```python
from build123d import *

# Parameters (mm, degrees)
F2_DEPTH = 40
F6_DEPTH = 40.001
F7_DEPTH = 40.001


with BuildPart() as f2:
    # F1 (on face) → F2 (new body)
    with BuildSketch(Plane.XY):
        Polygon((-30.25273, 38.586084), (-30.25273, 0), (-26.359774, 0), (-20, 11.340041), (-20, 0), (-10, 0), (-10, 11.340041), (0, 11.340041), (0, 0), (9.197158, 0), (9.197158, 11.045149), (13.475588, 0), (26.648319, 0), (34.74727, 11.808881), (34.74727, 38.586084), align=None)
        Polygon((-26.625307, 52.630479), (-42.740828, 52.770232), (-42.740828, 0), (-30.25273, 0), (-30.25273, 38.586084), (34.74727, 38.586084), (34.74727, 11.808881), (37.706377, 16.123482), (37.706377, 36.123482), (26.394449, 52.617125), (13.475588, 52.617125), (13.475588, 41.231845), (4.72787, 52.630479), (-15.074225, 52.630479), (-18.680247, 41.231845), (-22.642306, 48.647475), align=None)
    extrude(amount=F2_DEPTH)

    # F5 (on face) → F6 (cut, through all)
    with BuildSketch(Plane.XY.offset(40)):
        Polygon((-34.457395, 34.423446), (-34.457395, 24.423446), (-29.457395, 24.423446), (-29.457395, 29.423446), align=None)
        Polygon((25.539488, 27.917431), (20.539488, 32.917431), (20.539488, 22.917431), (25.539488, 22.917431), align=None)
    extrude(amount=-F6_DEPTH, mode=Mode.SUBTRACT)

    # F4 (on face) → F7 (cut, through all)
    with BuildSketch(Plane.XY.offset(40)):
        Polygon((-7.5, 36.869197), (-10, 27.186738), (0, 27.186738), (-2.5, 36.869197), align=None)
    extrude(amount=-F7_DEPTH, mode=Mode.SUBTRACT)


solid = f2.part
```
Here's how the part is built. I have some questions about the finished solid (model axes, mm). A direction names the side the tool comes from. Coordinates: 2 decimals unless noted, no trailing zeros. Order: outer loops, then holes, each group sorted by start corner. A loop starts at its lowest first (then second) coordinate and runs counter-clockwise, first axis right, second up.
1) Imagine slicing it at B-B on x = 8. List the corners of the cut face in (y, z) for me.
2) Imagine slicing it at A-A on z = 36.5. State how many separate pieces and enclosed holes the cut face has, and give its area (3 significant figures).
3) Which directions (+Z, -Z, +X, -X, +Y, -Y) give clear straight access to the entire face, cutting with the end or side of a thin tool? Please do faces 4 (the face through (9.163, 46.851, 19.72)), 5 (the face through (20.539, 28, 20)), 6 (the face through (-35, 0, 20)).
4) Imagine slicing it at C-C on y = 13. List the corners of the cut face in (x, z) for me.
5) I need wall thicknesses on line 1 (X direction, y = 49, z = 5.5); line 2 (Y direction, x = -3.5, z = 29.5); line 3 (X direction, y = 45, z = 32). Which ranges of each line are inside material? Lowest first, please.
6) Will these pins go through, and if not, where does the flat tip stop? pin 1 (11 mm diameter, centred on x = -7, z = 19, fed in from -Y); pin 2 (5.5 mm diameter, centred on x = 22, z = 13.5, fed in from +Y); pin 3 (9 mm diameter, centred on y = 7.5, z = 25.5, fed in from +X); pin 4 (2.5 mm diameter, centred on x = -33, z = 20, fed in from +Y).
7) We'd pull the mould along X, two halves only. Please class faces 1 (the face through (32.1, 44.3, 19.7)), 2 (the face through (-34.457, 29, 20)), 3 (the face through (-42.741, 27, 20)): +X half, -X half, draft (parallel to the pull), parting line (faces both ways), or undercut.
Response values:
1. outline: (0, 0) - (48.37, 0) - (48.37, 40) - (0, 40) - close
2. separate pieces: 1
2. enclosed holes: 3
2. area: 3,620 mm2
3. face 4: +Z, -Z, +Y
3. face 5: +Z, -Z
3. face 6: +Z, -Z, +X, -X, -Y
4. outline: (-42.74, 0) - (35.56, 0) - (35.56, 40) - (-42.74, 40) - close
5. line 1: x = -42.74 to -22.99, -16.22 to 7.51, 13.48 to 28.88
5. line 2: y = 11.34 to 27.19, 36.87 to 52.63
5. line 3: x = -42.74 to -20.69, -17.49 to 10.58, 13.48 to 31.62
6. pin 1: stops at y = 0
6. pin 2: stops at y = 52.62
6. pin 3: stops at x = 34.88
6. pin 4: stops at y = 52.7
7. face 1: +X half
7. face 2: undercut
7. face 3: -X half
